Work out the finished part from the listing and answer in its coordinate system (mm). Coordinates: 2 decimals unless noted, no trailing zeros. Order: outer loops, then holes, each group sorted by start corner. A loop starts at its lowest first (then second) coordinate and runs counter-clockwise, first axis right, second up. Notation, with made-up numbers: M 46.25,4.25 L 80.25,4.25 A12 ccw 80.25,17.25 Z; hole C 41,-35.5 d11. An arc over 180 degrees is marked long. Use a Markdown table: item, result.
from build123d import *

# Parameters (mm, degrees)
GENERICCARDPCBDEFINITION_START = -0.8
GENERICCARDPCBDEFINITION_DEPTH = 1.6
SKETCH7_R                      = 1.2
CUT_EXTRUDE1_DEPTH             = 71.516735602
FILLET1_R                      = 0.5


# Read off the part's stored shape, not the designer's step: GenericCardPCBDefinition
with BuildPart() as part:
    # GenericCardPCBDefinition outline → GenericCardPCBDefinition (new body)
    with BuildSketch(Plane(origin=(0, 0, 0), x_dir=(1, 0, 0), z_dir=(0, 1, 0)).offset(GENERICCARDPCBDEFINITION_START)):
        with BuildLine():
            Line((-49.9, -39), (-44.1, -44.8))
            Line((-44.1, -44.8), (-41.232050808, -44.8))
            ThreePointArc((-41.232050808, -44.8), (-39.5, -43.8), (-37.767949192, -44.8))
            Line((-37.767949192, -44.8), (-18.232050808, -44.8))
            ThreePointArc((-18.232050808, -44.8), (-16.5, -43.8), (-14.767949192, -44.8))
            Line((-14.767949192, -44.8), (14.767949192, -44.8))
            ThreePointArc((14.767949192, -44.8), (16.5, -43.8), (18.232050808, -44.8))
            Line((18.232050808, -44.8), (37.767949192, -44.8))
            ThreePointArc((37.767949192, -44.8), (39.5, -43.8), (41.232050808, -44.8))
            Line((41.232050808, -44.8), (44.1, -44.8))
            Line((44.1, -44.8), (49.9, -39))
            Line((49.9, -39), (49.9, 40.7))
            ThreePointArc((49.9, 40.7), (49.753553391, 41.053553391), (49.4, 41.2))
            Line((49.4, 41.2), (47.65, 41.2))
            ThreePointArc((47.65, 41.2), (47.296446609, 41.346446609), (47.15, 41.7))
            Line((47.15, 41.7), (47.15, 46.4))
            ThreePointArc((47.15, 46.4), (47.003553391, 46.753553391), (46.65, 46.9))
            Line((46.65, 46.9), (34.9, 46.9))
            ThreePointArc((34.9, 46.9), (34.546446609, 47.046446609), (34.4, 47.4))
            Line((34.4, 47.4), (34.4, 49.3))
            ThreePointArc((34.4, 49.3), (34.253553391, 49.653553391), (33.9, 49.8))
            Line((33.9, 49.8), (-33.9, 49.8))
            ThreePointArc((-33.9, 49.8), (-34.253553391, 49.653553391), (-34.4, 49.3))
            Line((-34.4, 49.3), (-34.4, 47.4))
            ThreePointArc((-34.4, 47.4), (-34.546446609, 47.046446609), (-34.9, 46.9))
            Line((-34.9, 46.9), (-46.65, 46.9))
            ThreePointArc((-46.65, 46.9), (-47.003553391, 46.753553391), (-47.15, 46.4))
            Line((-47.15, 46.4), (-47.15, 41.7))
            ThreePointArc((-47.15, 41.7), (-47.296446609, 41.346446609), (-47.65, 41.2))
            Line((-47.65, 41.2), (-49.4, 41.2))
            ThreePointArc((-49.4, 41.2), (-49.753553391, 41.053553391), (-49.9, 40.7))
            Line((-49.9, 40.7), (-49.9, -39))
        make_face()
    extrude(amount=GENERICCARDPCBDEFINITION_DEPTH)

    # Sketch7 → Cut-Extrude1 (cut, through all)
    with BuildSketch(Plane.XZ.offset(0.8)):
        with Locations(Location((3.9, -41.7, 0), (0, 0, 270))):
            Circle(SKETCH7_R)
        with Locations(Location((3.9, -30.1, 0), (0, 0, 270))):
            Circle(SKETCH7_R)
        with Locations(Location((43.65, -41.7, 0), (0, 0, 270))):
            Circle(SKETCH7_R)
        with Locations(Location((43.65, -30.1, 0), (0, 0, 270))):
            Circle(SKETCH7_R)
        with BuildLine():
            Line((38.65, -20.9), (8.9, -20.9))
            ThreePointArc((8.9, -20.9), (7.485786438, -21.485786438), (6.9, -22.9))
            Line((6.9, -22.9), (6.9, -49.8))
            Line((6.9, -49.8), (40.65, -49.8))
            Line((40.65, -49.8), (40.65, -22.9))
            ThreePointArc((40.65, -22.9), (40.064213562, -21.485786438), (38.65, -20.9))
        make_face()
    extrude(amount=-CUT_EXTRUDE1_DEPTH, mode=Mode.SUBTRACT)

    # Fillet1
    fillet1_edges = [part.edges().sort_by_distance(p)[0] for p in [
        (40.65, 0, -46.9),
        (6.9, 0, -49.8),
    ]]
    fillet(fillet1_edges, radius=FILLET1_R)


solid = part.part
1. Section A-A on z = -24.5 is taken. Determine the outline of the cut face in (x, y), then the cut area to 3 significant figures.
Answers below:
| item | result |
|---|---|
| outline | M -49.9,-0.8 L 6.9,-0.8 L 6.9,0.8 L -49.9,0.8 Z; M 40.65,-0.8 L 49.9,-0.8 L 49.9,0.8 L 40.65,0.8 Z |
| area | 106 mm² |
2. Find the intervals of material crossed by probe 1 along X at (y, z) = (0, -41.7); probe 2 along X at (y, z) = (-0.4, -30.1); probe 3 along X at (y, z) = (-0.05, -32.5), in increasing order.
Answers below:
| item | result |
|---|---|
| probe 1 | -47.15 to 2.7, 5.1 to 6.9, 40.65 to 42.45, 44.85 to 47.15 |
| probe 2 | -49.9 to 2.7, 5.1 to 6.9, 40.65 to 42.45, 44.85 to 49.9 |
| probe 3 | -49.9 to 6.9, 40.65 to 49.9 |
3. Flat-ended cylindrical pins translate along their axes: P1, Ø0.5, axis at x = 43.5, y = 0, coming from the -Z side; P2, Ø4, axis at x = 43.65, z = -41.7, coming from the -Y side; P3, Ø1.9, axis at x = 3.9, z = -30.1, coming from the -Y side; P4, Ø0.5, axis at y = 0, z = -48, coming from the -X side. Find the tip coordinate at first contact, or state that the pin passes through.
Answers below:
| item | result |
|---|---|
| P1 | z = -46.9 |
| P2 | y = -0.8 |
| P3 | through |
| P4 | x = -34.4 |
4. Section B-B on x = 3.9 is taken. Determine the outline of the cut face in (y, z).
Answers below:
| item | result |
|---|---|
| outline | M -0.8,-49.8 L 0.8,-49.8 L 0.8,-42.9 L -0.8,-42.9 Z; M -0.8,-40.5 L 0.8,-40.5 L 0.8,-31.3 L -0.8,-31.3 Z; M -0.8,-28.9 L 0.8,-28.9 L 0.8,44.8 L -0.8,44.8 Z |
5. For a pull along Z with two mould halves and no side action, classify faces 1 (the face through (-1, 0.8, -3)), 2 (the face through (47, 0, 41.9)), 3 (the face through (3.95, -0.01, -40.5)) as +Z half, -Z half, draft (parallel to the pull), parting line (faces both ways), or undercut.
Answers below:
| item | result |
|---|---|
| face 1 | draft |
| face 2 | +Z half |
| face 3 | undercut |
6. Section C-C on y = 0.2 is taken. Give the number of separate pieces and of enclosed holes in the cut face, then the cut area to 3 significant figures.
Answers below:
| item | result |
|---|---|
| separate pieces | 1 |
| enclosed holes | 4 |
| area | 8,300 mm² |
